Here's how the part is built. I have some questions about the finished solid (model axes, mm). Coordinates: 2 decimals unless noted, no trailing zeros. Write each loop counter-clockwise with the first axis right and the second up, starting at its lowest first coordinate (ties: lowest second). Pieces come first, ordered by that corner, then holes. Notation, with made-up numbers: M -18,20.25 L -1,20.25 A22 cw -1,46.25 Z; hole C 49.5,61 d2. An arc over 180 degrees is marked long. Use a Markdown table: item, result.
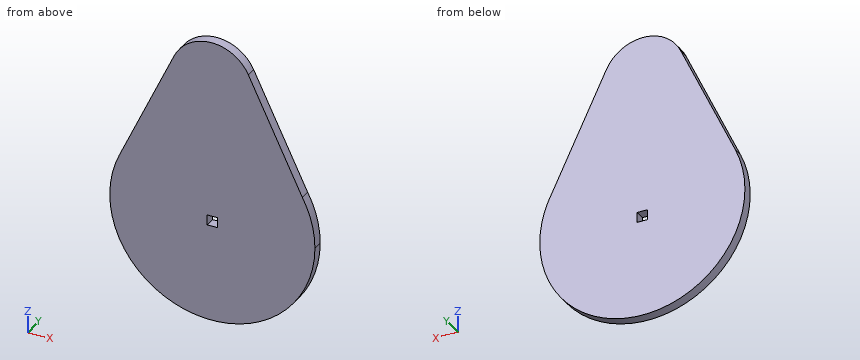
```python
from build123d import *

# Parameters (mm, degrees)
F0_W     = 3.175
F0_H     = 3.175
F1_DEPTH = 3.175


with BuildPart() as f1:
    # F0 (on Front) → F1 (new body)
    with BuildSketch(Plane.XZ):
        with BuildLine():
            ThreePointArc((-73.961423, 42.131236), (-52.05154, -2.278535), (-13.433104, 28.719644))
            ThreePointArc((-13.433104, 28.719644), (-14.429342, 36.610694), (-17.35554, 44.00654))
            ThreePointArc((-17.35554, 44.00654), (-46.234377, 60.452235), (-73.961423, 42.131236))
        make_face()
        with Locations((-45.183104, 28.719644)):
            Rectangle(F0_W, F0_H, mode=Mode.SUBTRACT)
        with BuildLine():
            ThreePointArc((-73.961423, 42.131236), (-46.234377, 60.452235), (-17.35554, 44.00654))
            Line((-17.35554, 44.00654), (-34.04271, 78.677435))
            ThreePointArc((-34.04271, 78.677435), (-33.104337, 75.99429), (-32.786234, 73.169644))
            ThreePointArc((-32.786234, 73.169644), (-48.156231, 60.753481), (-57.063575, 78.390292))
            Line((-57.063575, 78.390292), (-73.961423, 42.131236))
        make_face()
        with BuildLine():
            ThreePointArc((-32.786234, 73.169644), (-33.104337, 75.99429), (-34.04271, 78.677435))
            Line((-34.04271, 78.677435), (-56.929758, 78.677435))
            Line((-56.929758, 78.677435), (-57.063575, 78.390292))
            ThreePointArc((-57.063575, 78.390292), (-48.156231, 60.753481), (-32.786234, 73.169644))
        make_face()
        with BuildLine():
            Line((-56.929758, 78.677435), (-34.04271, 78.677435))
            ThreePointArc((-34.04271, 78.677435), (-45.486234, 85.869644), (-56.929758, 78.677435))
        make_face()
    extrude(amount=F1_DEPTH)


solid = f1.part
```
1. Suppose I cut it at A-A on y = -2.5. Write out the boundary of the cut face in (x, z).
Answers follow:
| item | result |
|---|---|
| outline | M -73.96,42.13 A31.75 ccw long -13.43,28.72 A31.75 ccw -17.36,44.01 L -34.04,78.68 A12.7 ccw -56.93,78.68 L -57.06,78.39 Z; hole M -46.77,27.13 L -43.6,27.13 L -43.6,30.31 L -46.77,30.31 Z |
2. Suppose I cut it at D-D on x = -37. Write out the boundary of the cut face in (y, z) (3 decimals), and give its area (3 significant figures).
Answers follow:
| item | result |
|---|---|
| outline | M -3.175,-1.958 L 0,-1.958 L 0,82.618 L -3.175,82.618 Z |
| area | 269 mm2 |
3. Will these pins go through, and if not, where does the flat tip stop? pin 1 Ø1 at (y, z) = (-0.5, 10.5) entering from +X; pin 2 Ø1 at (y, z) = (-0.5, 67.5) entering from +X.
Answers follow:
| item | result |
|---|---|
| pin 1 | stops at x = -18.84 |
| pin 2 | stops at x = -28.42 |
4. Suppose I cut it at B-B on x = -44.5. Write out the boundary of the cut face in (y, z) (3 decimals).
Answers follow:
| item | result |
|---|---|
| outline | M -3.175,-3.023 L 0,-3.023 L 0,27.132 L -3.175,27.132 Z; M -3.175,30.307 L 0,30.307 L 0,85.831 L -3.175,85.831 Z |
5. I need wall thicknesses on probe 1 along X at (y, z) = (-1.05, 78); probe 2 along Z at (x, y) = (-71, -0.2); probe 3 along Z at (x, y) = (-29, -0.15). Which ranges of each line are inside material? Lowest first, please.
Answers follow:
| item | result |
|---|---|
| probe 1 | x = -57.25 to -33.72 |
| probe 2 | z = 10.24 to 48.49 |
| probe 3 | z = 1.4 to 68.2 |
6. Suppose I cut it at C-C on z = 19. Write out the boundary of the cut face in (x, y) (3 decimals), and give its area (3 significant figures).
Answers follow:
| item | result |
|---|---|
| outline | M -75.409,-3.175 L -14.957,-3.175 L -14.957,0 L -75.409,0 Z |
| area | 192 mm2 |
